```python
from build123d import *

# Parameters (mm, degrees)
F0_W     = 14
F0_H     = 14
F1_DEPTH = 60
F3_DEPTH = 25
F5_DEPTH = 25


with BuildPart() as f1:
    # F0 (on Top) → F1 (new body)
    with BuildSketch(Plane.XY):
        Rectangle(F0_W, F0_H)
    extrude(amount=F1_DEPTH)

    # F2 (on face) → F3 (cut)
    with BuildSketch(Plane.XZ.offset(7)):
        Polygon((-7, 46), (7, 60), (-7, 60), align=None)
    extrude(amount=-F3_DEPTH, mode=Mode.SUBTRACT)

    # F4 (on face) → F5 (cut)
    with BuildSketch(Plane.XZ.offset(7)):
        Polygon((-7, 0), (7, 0), (-7, 14), align=None)
    extrude(amount=-F5_DEPTH, mode=Mode.SUBTRACT)


solid = f1.part
```
Geometry check sheet. Reference: the model listing, model coordinates, mm. Coordinates: 2 decimals unless noted, no trailing zeros. Loops run counter-clockwise (first coordinate to the right, second up) from the corner with the lowest first, then second, coordinate; pieces in that order, holes last. Notation, with made-up numbers: (69, 1) -> (88, 1) arc R14 cw to (88, 5) -> close; hole circle Ø1 at (-14.75, 86). An arc over 180 degrees is marked (long way). Put each result on its own line as item: value.
1) Thickness scan on line 1 (X direction, y = 2.25, z = 55); line 2 (Z direction, x = -2, y = -2); line 3 (Z direction, x = 0, y = -4.5). Record the ranges inside material, lowest first.
Result set:
line 1: x = 2 to 7
line 2: z = 9 to 51
line 3: z = 7 to 53
2) Cross-section at B-B on z = 47. Record the boundary of the cut face in (x, y).
Result set:
outline: (-6, -7) -> (7, -7) -> (7, 7) -> (-6, 7) -> close
3) Gauge pin test, flat ends, axial feed: pin 1 Ø8 at (x, y) = (0.5, 5) entering from +Z; pin 2 Ø4 at (y, z) = (4.5, 53.5) entering from -X; pin 3 Ø1.5 at (x, y) = (-2.5, -1.5) entering from +Z. Record the tip position at first contact, or that the pin passes through.
Result set:
pin 1: stops at z = 57.5
pin 2: stops at x = -1.5
pin 3: stops at z = 51.25
4) Cross-section at A-A on x = -2.5. Record the boundary of the cut face in (y, z), plus the area to 3 significant figures.
Result set:
outline: (-7, 9.5) -> (7, 9.5) -> (7, 50.5) -> (-7, 50.5) -> close
area: 574 mm^2
